Could you check a few things on this model? Use its own coordinates, in mm. A direction names the side the tool comes from. Coordinates: 2 decimals unless noted, no trailing zeros. Write each loop counter-clockwise with the first axis right and the second up, starting at its lowest first coordinate (ties: lowest second). Pieces come first, ordered by that corner, then holes. Notation, with made-up numbers: (52.5, -19.75) - (86.5, -19.75) arc R23 cw to (86.5, 17.25) - close; hole circle Ø9 at (-30.5, 46.5). An arc over 180 degrees is marked (long way). Answer as a JSON object with one key per item and string values. Group by question number.
1) If we section it at A-A (z = 30): Write out the boundary of the cut face in (x, y), plus the area to 3 significant figures.
2) Will these pins go through, and if not, where does the flat tip stop? pin 1 Ø18 at (y, z) = (-6, 64.5) entering from -X; pin 2 Ø4 at (x, y) = (47, -7) entering from +Z; pin 3 Ø4 at (x, y) = (66.5, 0.5) entering from +Z.
3) We'd pull the mould along Y, two halves only. Please class faces 5 (the cylindrical face through (57, 29, 88)), 6 (the flat face through (25, 0, 20)), 7 (the flat face through (59, 0, 75)): released by +Y, released by -Y, zero draft, split by the parting line, or undercut.
4) If we section it at C-C (y = -20): Write out the boundary of the cut face in (x, z), plus the area to 3 significant figures.
5) On a 3-axis mill with a long thin cutter (end or side, diameter ignored), from which of +Z, -Z, +X, -X, +Y, -Y can I reach the whole of each face in a straight line? I mean faces 1 (the flat face through (50, 0, 55)), 2 (the flat face through (93, 0, 20)), 3 (the flat face through (52, -19, 28)), 4 (the flat face through (62, 10, 80)). Say none if no direction works.
6) If we section it at D-D (x = 43.5): Write out the boundary of the cut face in (y, z).
7) Please list where these lines run through material, in increasing order: line 1 along Y through (x, z) = (67, 30); line 2 along Y through (x, z) = (60, 80); line 3 along Z through (x, y) = (60.5, -20).
```python
from build123d import *

# Parameters (mm, degrees)
F1_DEPTH       = 30
F2_R           = 29.99999
F4_D           = 3.4
F4_CBORE_D     = 7
F4_CBORE_DEPTH = 2
F5_SIZE        = 8
F10_DEPTH      = 16
F11_DEPTH      = 60.001
F12_R          = 5


# Not quite as in the source:
# - a fillet or chamfer is up to 0.001 mm smaller than in the source, because OpenCascade refuses the exact size


with BuildPart() as f1:
    # F0 (on Front) → F1 (new body, symmetric)
    with BuildSketch(Plane.XZ):
        Polygon((0, 20), (0, 0), (120, 0), (120, 20), (75, 20), (75, 90), (50, 90), (50, 20), align=None)
    extrude(amount=F1_DEPTH, both=True)

    # F2 (radius 30 in the source; OpenCascade refuses exactly that, so slightly less here)
    f2_edges = [f1.edges().sort_by_distance(p)[0] for p in [
        (120, -30, 10),
        (120, 30, 10),
    ]]
    fillet(f2_edges, radius=F2_R)

    # F4 (through all)
    with Locations(Plane(origin=(50, 0, 0), x_dir=(0, -1, 0), z_dir=(-1, 0, 0))):
        with Locations((-20, 80), (-20, 30), (20, 30), (20, 80)):
            CounterBoreHole(F4_D / 2, F4_CBORE_D / 2, F4_CBORE_DEPTH)

    # F5
    f5_edges = [f1.edges().sort_by_distance(p)[0] for p in [
        (0, 30, 10),
        (0, -30, 10),
    ]]
    chamfer(f5_edges, length=F5_SIZE)

    # F7 (on face) → F10 (cut, through all)
    with BuildSketch(Plane.YZ.offset(75)):
        with BuildLine():
            ThreePointArc((-10, 70), (0, 80), (10, 70))
            Line((10, 70), (10, 90))
            Line((10, 90), (-10, 90))
            Line((-10, 90), (-10, 70))
        make_face()
        with BuildLine():
            ThreePointArc((-10, 70), (0, 60), (10, 70))
            ThreePointArc((10, 70), (0, 80), (-10, 70))
        make_face()
    extrude(amount=-F10_DEPTH, mode=Mode.SUBTRACT)

    # F6 (on face) → F11 (cut, through all)
    with BuildSketch(Plane.XZ.offset(30)):
        Polygon((62.6571113504, 90), (75, 20), (75, 90), align=None)
    extrude(amount=-F11_DEPTH, mode=Mode.SUBTRACT)

    # F12
    f12_edges = [f1.edges().sort_by_distance(p)[0] for p in [
        (56.328556, -30, 90),
        (56.328556, 30, 90),
    ]]
    fillet(f12_edges, radius=F12_R)


solid = f1.part
```
Here are the results:
{
 "1": {"outline": "(50, -30) - (73.24, -30) - (73.24, -21.7) - (52, -21.7) - (52, -23.5) - (50, -23.5) - close; (50, -16.5) - (52, -16.5) - (52, -18.3) - (73.24, -18.3) - (73.24, 18.3) - (52, 18.3) - (52, 16.5) - (50, 16.5) - close; (50, 23.5) - (52, 23.5) - (52, 21.7) - (73.24, 21.7) - (73.24, 30) - (50, 30) - close", "area": "1,220 mm²"},
 "2": {"pin 1": "stops at x = 50", "pin 2": "stops at z = 20", "pin 3": "stops at z = 60.32"},
 "3": {"face 5": "released by +Y", "face 6": "zero draft", "face 7": "undercut"},
 "4": {"outline": "(0, 0) - (112.36, 0) - (112.36, 20) - (75, 20) - (73.54, 28.3) - (52, 28.3) - (52, 26.5) - (50, 26.5) - (50, 20) - (0, 20) - close; (50, 33.5) - (52, 33.5) - (52, 31.7) - (72.94, 31.7) - (64.72, 78.3) - (52, 78.3) - (52, 76.5) - (50, 76.5) - close; (50, 83.5) - (52, 83.5) - (52, 81.7) - (64.12, 81.7) - (62.66, 90) - (50, 90) - close", "area": "3,420 mm²"},
 "5": {"face 1": "+Z, -X, +Y, -Y", "face 2": "+Z, +X, +Y, -Y", "face 3": "-X", "face 4": "+Z, +X"},
 "6": {"outline": "(-30, 0) - (30, 0) - (30, 20) - (-30, 20) - close"},
 "7": {"line 1": "y = -30 to -21.7, -18.3 to 18.3, 21.7 to 30", "line 2": "y = -30 to -21.7, -18.3 to -10, 10 to 18.3, 21.7 to 30", "line 3": "z = 0 to 28.3, 31.7 to 78.3, 81.7 to 90"}
}
